Model file for the job. Use its own axes, mm. A direction names the side the tool comes from. Coordinates: 2 decimals unless noted, no trailing zeros. Order: outer loops, then holes, each group sorted by start corner. A loop starts at its lowest first (then second) coordinate and runs counter-clockwise, first axis right, second up. Notation, with made-up numbers: (14, 59.25) -> (52, 59.25) arc R19 cw to (52, 65.25) -> close; hole circle Ø2 at (56, -6.75). An arc over 180 degrees is marked (long way). Use CSV: the item, a comma, the result in double quotes. Start each with the question number.
(1) Pin check, flat tips, straight feed: pin 1 Ø0.8 at (x, y) = (-0.5, -0.5) entering from +Z; pin 2 Ø4 at (x, z) = (-3, 19.5) entering from -Y. Stop position of each tip, or through.
(2) Tool access for faces 4 (the cylindrical face through (0, 2, 11)), 5 (the flat face through (0, 0, 0)), 6 (the flat face through (0, 0, 23.5)): list every direction of +Z, -Z, +X, -X, +Y, -Y with a clear straight run to the whole face (end or side of a thin tool).
(3) Cut at B-B on z = 2.5. Write the cut outline in (x, y), plus the area to 3 significant figures.
(4) Cut at A-A on x = 0. Write the cut outline in (y, z), plus the area to 3 significant figures.
(5) Pull direction Y, two halves, no side cores. Call faces 1 (the flat face through (-0.125, 1.244, 24.26)), 2 (the flat face through (0, -2, 25)), 3 (the conical face through (2.045, 0.644, 22.664)): pulls with the +Y half, pulls with the -Y half, needs draft (parallel to the pull), parting line crosses it, or undercut.
(6) Probe L1, parallel to Y at x = 0, z = 12; L2, parallel to Z at x = -0.75, y = 0; L3, parallel to Y at x = -0.5, z = 24.25. List the from-to ranges inside material, lowest first.
Autodesk Inventor part; units mm, degrees
ref_plane "YZ Plane" through (0, 0, 0) normal (1, 0, 0) x (0, 1, 0)
ref_plane "XZ Plane" through (0, 0, 0) normal (0, 1, 0) x (-1, 0, 0)
ref_plane "XY Plane" through (0, 0, 0) normal (0, 0, 1) x (1, 0, 0)
sketch "Sketch1" plane through (0, 0, 0) normal (0, 0, 1) x (1, 0, 0)
  circle A0 centre (0, 0) radius 2
  dimension "Diameter" = 4
extrude "Extrusion1" add sketch "Sketch1" along normal blind 22.52
sketch "Sketch2" plane through (0, 0, 22.52) normal (0, 0, 1) x (1, 0, 0)
  circle A0 centre (0, 0) radius 2
extrude "Extrusion2" add sketch "Sketch2" along normal blind 2.48 draft 45
sketch "Sketch3" plane through (0, 0, 25) normal (0, 0, 1) x (1, 0, 0)
  circle A0 centre (0, 0) radius 4.48
  circle A1 centre (0, 0) radius 1.4434 construction
  line L0 (0.6042, 1.3108) -> (1.4373, 0.1322)
  line L1 (1.4373, 0.1322) -> (0.8331, -1.1787)
  line L2 (0.8331, -1.1787) -> (-0.6042, -1.3108)
  line L3 (-0.6042, -1.3108) -> (-1.4373, -0.1322)
  line L4 (-1.4373, -0.1322) -> (-0.8331, 1.1787)
  line L5 (-0.8331, 1.1787) -> (0.6042, 1.3108)
  dimension "Hex_Width" = 2.5
extrude "Extrusion3" cut sketch "Sketch3" against normal blind 1.5 contours L0 L1 L2 L3 L4 L5
thread "Thread1"
chamfer "Chamfer2" distance 0.4 angle 45 1 edges at (-2, 0, 0)
fillet "Fillet1" radius 0.1 1 edges at (-4.48, 0, 25)
equation "\"d10\" = Thread_Length"
equation "\"d13\" = Chamfer"
equation "\"Thread_Length\" = 7.52"
properties part number "SCREW, FLAT HD, P, 12_9, M4X0_7X25"
Outcome:
1,pin 1,"z = 23.5"
1,pin 2,"y = -1.73"
2,face 4,"-Z"
2,face 5,"-Z, +X, -X, +Y, -Y"
2,face 6,"+Z"
3,outline,"circle Ø4 at (0, 0)"
3,area,"12.6 mm2"
4,outline,"(-4.31, 24.83) -> (-2, 22.52) -> (-2, 0.4) -> (-1.6, 0) -> (1.6, 0) -> (2, 0.4) -> (2, 22.52) -> (4.31, 24.83) arc R0.1 ccw to (4.24, 25) -> (1.26, 25) -> (1.26, 23.5) -> (-1.26, 23.5) -> (-1.26, 25) -> (-4.24, 25) arc R0.1 ccw to start"
4,area,"102 mm2"
5,face 1,"undercut"
5,face 2,"needs draft"
5,face 3,"parting line crosses it"
6,L1,"-2 to 2"
6,L2,"0 to 23.5"
6,L3,"-3.7 to -1.3, 1.21 to 3.7"
